from build123d import *

# Parameters (mm, degrees)
F0_W     = 76.2
F0_H     = 50.8
F1_DEPTH = 12.7
F2_R     = 6.35
F3_DEPTH = 25.4
F4_R     = 6.35
F5_DEPTH = 76.2
F6_R     = 6.35
F7_DEPTH = 50.8


with BuildPart() as f1:
    # F0 (on Front) → F1 (new body, symmetric)
    with BuildSketch(Plane.XZ):
        Rectangle(F0_W, F0_H)
    extrude(amount=F1_DEPTH, both=True)

    # F2 (on face) → F3 (cut, through all)
    with BuildSketch(Plane.XZ.offset(12.7)):
        with Locations((-25.4, 12.7)):
            Circle(F2_R)
        with Locations((0, 12.7)):
            Circle(F2_R)
        with Locations((25.4, 12.7)):
            Circle(F2_R)
        with Locations((-25.4, -12.7)):
            Circle(F2_R)
        with Locations((0, -12.7)):
            Circle(F2_R)
        with Locations((25.4, -12.7)):
            Circle(F2_R)
    extrude(amount=-F3_DEPTH, mode=Mode.SUBTRACT)

    # F4 (on face) → F5 (cut, through all)
    with BuildSketch(Plane(origin=(-38.1, 0, 0), x_dir=(0, -1, 0), z_dir=(-1, 0, 0))):
        with Locations((0, 12.7)):
            Circle(F4_R)
        with Locations((0, -12.7)):
            Circle(F4_R)
    extrude(amount=-F5_DEPTH, mode=Mode.SUBTRACT)

    # F6 (on face) → F7 (cut, through all)
    with BuildSketch(Plane(origin=(0, 0, -25.4), x_dir=(1, 0, 0), z_dir=(0, 0, -1))):
        with Locations((-25.4, 0)):
            Circle(F6_R)
        Circle(F6_R)
        with Locations((25.4, 0)):
            Circle(F6_R)
    extrude(amount=-F7_DEPTH, mode=Mode.SUBTRACT)


solid = f1.part
Could you check a few things on this model? Use its own coordinates, in mm. Give positions to 0.01 mm unless a question says otherwise; leave off trailing zeros. Order: outer loops, then holes, each group sorted by start corner. A loop starts at its lowest first (then second) coordinate and runs counter-clockwise, first axis right, second up.
1. Suppose I cut it at A-A (x = -25.4). List the corners of the cut face in (y, z) for me.
2. Suppose I cut it at B-B (z = 22.5). List the corners of the cut face in (x, y) for me.
3. Suppose I cut it at D-D (z = 12.7). Give the number of separate pieces and of enclosed holes in the cut face, plus the area to 3 significant figures.
4. We'd pull the mould along X, two halves only. Please class faces 1 (the cylindrical face through (20.72, 9.45, 16.99)), 2 (the flat face through (38.1, 0, 0)), 3 (the cylindrical face through (12.585, 6.344, -12.421)): pulls with the +X half, pulls with the -X half, needs draft (parallel to the pull), parting line crosses it, or undercut.
5. I need wall thicknesses on L1, parallel to Z at x = 4.5, y = 6; L2, parallel to X at y = 0, z = 1.5; L3, parallel to Z at x = 0, y = -7. Which ranges of each line are inside material? Lowest first, please.
6. Will this pin go through, and if not, where does the flat tip stop? P1, Ø10, axis at x = 25.4, z = 12.7, coming from the -Y side.
7. Suppose I cut it at C-C (y = 10). List the corners of the cut face in (x, z) for me, plus the area to 3 significant figures.
Solved:
1. outline: (-12.7, -25.4) - (-6.35, -25.4) - (-6.35, -19.05) - (-12.7, -19.05) - close; (-12.7, -6.35) - (-6.35, -6.35) - (-6.35, 6.35) - (-12.7, 6.35) - close; (-12.7, 19.05) - (-6.35, 19.05) - (-6.35, 25.4) - (-12.7, 25.4) - close; (6.35, -25.4) - (12.7, -25.4) - (12.7, -19.05) - (6.35, -19.05) - close; (6.35, -6.35) - (12.7, -6.35) - (12.7, 6.35) - (6.35, 6.35) - close; (6.35, 19.05) - (12.7, 19.05) - (12.7, 25.4) - (6.35, 25.4) - close
2. outline: (-38.1, -12.7) - (38.1, -12.7) - (38.1, 12.7) - (-38.1, 12.7) - close; hole circle Ø12.7 at (-25.4, 0); hole circle Ø12.7 at (0, 0); hole circle Ø12.7 at (25.4, 0)
3. separate pieces: 8
3. enclosed holes: 0
3. area: 484 mm2
4. face 1: undercut
4. face 2: pulls with the +X half
4. face 3: needs draft
5. L1: z = -25.4 to -17.18, -8.22 to 8.22, 17.18 to 25.4
5. L2: x = -38.1 to -31.75, -19.05 to -6.35, 6.35 to 19.05, 31.75 to 38.1
5. L3: z = -25.4 to -19.05, -6.35 to 6.35, 19.05 to 25.4
6. P1: passes through
7. outline: (-38.1, -25.4) - (38.1, -25.4) - (38.1, 25.4) - (-38.1, 25.4) - close; hole circle Ø12.7 at (-25.4, -12.7); hole circle Ø12.7 at (-25.4, 12.7); hole circle Ø12.7 at (0, -12.7); hole circle Ø12.7 at (0, 12.7); hole circle Ø12.7 at (25.4, -12.7); hole circle Ø12.7 at (25.4, 12.7)
7. area: 3,110 mm2
